from build123d import *

# Parameters (mm, degrees)
F0_W     = 127
F0_H     = 76.2
F1_DEPTH = 12.7
F3_D     = 12.7
F5_D     = 12.7
F7_D     = 12.7
F9_D     = 12.7
F10_W    = 12.7
F10_H    = 50.8
F12_W    = 17.789466
F12_H    = 19.05
F14_W    = 15.24
F14_H    = 12.7
F16_R    = 2.54
F17_SIZE = 5.08


with BuildPart() as f1:
    # F0 (on Top) → F1 (new body)
    with BuildSketch(Plane.XY):
        Rectangle(F0_W, F0_H)
    extrude(amount=F1_DEPTH)

    # F3 (through all)
    with Locations(Plane.XY.offset(12.7)):
        with Locations((-50.8, 25.4)):
            Hole(F3_D / 2)

    # F5 (through all)
    with Locations(Plane.XY.offset(12.7)):
        with Locations((50.8, 25.4)):
            Hole(F5_D / 2)

    # F7 (through all)
    with Locations(Plane.XY.offset(12.7)):
        with Locations((-50.8, -25.4)):
            Hole(F7_D / 2)

    # F9 (through all)
    with Locations(Plane.XY.offset(12.7)):
        with Locations((50.8, -25.4)):
            Hole(F9_D / 2)

    # F10 (on Front) → F11 (revolve)
    with BuildSketch(Plane.XZ):
        with Locations((6.35, 38.1)):
            Rectangle(F10_W, F10_H)
    revolve(axis=Axis((0, 0, 38.1), (0, 0, 1)))

    # F12 (on Front) → F13 (revolve)
    with BuildSketch(Plane.XZ):
        with Locations((8.894733, 22.225)):
            Rectangle(F12_W, F12_H)
    revolve(axis=Axis((0, 0, 22.225), (0, 0, -1)))

    # F14 (on Front) → F15 (revolve)
    with BuildSketch(Plane.XZ):
        with Locations((7.62, 57.15)):
            Rectangle(F14_W, F14_H)
    revolve(axis=Axis((0, 0, 57.15), (0, 0, -1)))

    # F16
    f16_edges = [f1.edges().sort_by_distance(p)[0] for p in [
        (-15.24, 0, 63.5),
        (-17.789466, 0, 12.7),
    ]]
    fillet(f16_edges, radius=F16_R)

    # F17
    f17_edges = [f1.edges().sort_by_distance(p)[0] for p in [
        (-63.5, 0, 12.7),
        (63.5, 0, 12.7),
        (0, -38.1, 12.7),
        (0, 38.1, 12.7),
    ]]
    chamfer(f17_edges, length=F17_SIZE)


solid = f1.part
Check sheet for the modelled part. Datum: model origin and axes. Units: mm. A direction names the side the tool comes from. Round coordinates to 2 decimals unless told otherwise and drop trailing zeros. Order: outer loops, then holes, each group sorted by start corner. A loop starts at its lowest first (then second) coordinate and runs counter-clockwise, first axis right, second up.
Q1. Set-up check for faces 1 (the face through (-0.89, 35.6, 10.12)), 2 (the face through (-2.75, -12.4, 41.41)), 3 (the face through (-13.112, -12.023, 23.611)): record each of +Z, -Z, +X, -X, +Y, -Y from which the full face is reachable in a straight line by a thin tool's end or side.
Filled sheet:
face 1: +Z, +X, -X, +Y
face 2: none
face 3: +Z
Q2. Depth check by flat-ended pin: P1, Ø15, axis at x = -6.5, y = -0.5, coming from the -Z side; P2, Ø16.5, axis at x = 50.8, y = 25.4, coming from the +Z side; P3, Ø10, axis at y = -2.5, z = 44.5, coming from the -X side; P4, Ø3, axis at y = -8.5, z = 40, coming from the -X side. Enter the tip coordinate at first touch or a pass-through.
Filled sheet:
P1: stops at z = 0
P2: stops at z = 12.7
P3: stops at x = -12.7
P4: stops at x = -10.6
Q3. Cross-section at D-D, the plane y = 0. Enter the section's corners in (x, z), plus the area to 3 significant figures.
Filled sheet:
outline: (-63.5, 0) - (63.5, 0) - (63.5, 7.62) - (58.42, 12.7) - (20.33, 12.7) arc R2.54 cw to (17.79, 15.24) - (17.79, 31.75) - (12.7, 31.75) - (12.7, 50.8) - (15.24, 50.8) - (15.24, 60.96) arc R2.54 ccw to (12.7, 63.5) - (-12.7, 63.5) arc R2.54 ccw to (-15.24, 60.96) - (-15.24, 50.8) - (-12.7, 50.8) - (-12.7, 31.75) - (-17.79, 31.75) - (-17.79, 15.24) arc R2.54 cw to (-20.33, 12.7) - (-58.42, 12.7) - (-63.5, 7.62) - close
area: 3,140 mm2
Q4. Cross-section at A-A, the plane x = -50.8. Enter the section's corners in (y, z), plus the area to 3 significant figures.
Filled sheet:
outline: (-38.1, 0) - (-31.75, 0) - (-31.75, 12.7) - (-33.02, 12.7) - (-38.1, 7.62) - close; (-19.05, 0) - (19.05, 0) - (19.05, 12.7) - (-19.05, 12.7) - close; (31.75, 0) - (38.1, 0) - (38.1, 7.62) - (33.02, 12.7) - (31.75, 12.7) - close
area: 619 mm2
Q5. Cross-section at B-B, the plane y = -25.4. Enter the section's corners in (x, z).
Filled sheet:
outline: (-63.5, 0) - (-57.15, 0) - (-57.15, 12.7) - (-58.42, 12.7) - (-63.5, 7.62) - close; (-44.45, 0) - (44.45, 0) - (44.45, 12.7) - (-44.45, 12.7) - close; (57.15, 0) - (63.5, 0) - (63.5, 7.62) - (58.42, 12.7) - (57.15, 12.7) - close
Q6. Cross-section at C-C, the plane x = 0. Enter the section's corners in (y, z), plus the area to 3 significant figures.
Filled sheet:
outline: (-38.1, 0) - (38.1, 0) - (38.1, 7.62) - (33.02, 12.7) - (20.33, 12.7) arc R2.54 cw to (17.79, 15.24) - (17.79, 31.75) - (12.7, 31.75) - (12.7, 50.8) - (15.24, 50.8) - (15.24, 60.96) arc R2.54 ccw to (12.7, 63.5) - (-12.7, 63.5) arc R2.54 ccw to (-15.24, 60.96) - (-15.24, 50.8) - (-12.7, 50.8) - (-12.7, 31.75) - (-17.79, 31.75) - (-17.79, 15.24) arc R2.54 cw to (-20.33, 12.7) - (-33.02, 12.7) - (-38.1, 7.62) - close
area: 2,490 mm2
Q7. Draft check along Y on faces 4 (the face through (-61, -0.53, 10.12)), 5 (the face through (-56.666, -27.832, 6.261)), 6 (the face through (-3.3, 14.88, 55.95)). Enter one of: pulls with the +Y half, pulls with the -Y half, needs draft (parallel to the pull), parting line crosses it, or undercut.
Filled sheet:
face 4: needs draft
face 5: undercut
face 6: parting line crosses it
Q8. Scan lines: L1, parallel to X at y = -25, z = 7; L2, parallel to Y at x = -50.8, z = 3.5; L3, parallel to Y at x = -49, z = 4.5. Record each from-to range of solid material in increasing order.
Filled sheet:
L1: x = -63.5 to -57.14, -44.46 to 44.46, 57.14 to 63.5
L2: y = -38.1 to -31.75, -19.05 to 19.05, 31.75 to 38.1
L3: y = -38.1 to -31.49, -19.31 to 19.31, 31.49 to 38.1
